Job drawing, mm, ordinate dimensions from the low corner. One solid piece. A direction names the side the tool comes from. Coordinates: 2 decimals unless noted, no trailing zeros. Write each loop counter-clockwise with the first axis right and the second up, starting at its lowest first coordinate (ties: lowest second). Pieces come first, ordered by that corner, then holes. Notation, with made-up numbers: (29, 54) - (49, 54) arc R14 ccw to (49, 78) - close; hole circle Ø4 at (36, 24.5). An arc over 180 degrees is marked (long way). Put each result on its own line as item: value. Start each with the question number.
1. Saw through at D-D, the plane y = 2.5. Write the cut outline in (x, z).
2. Drop flat-ended pins along their axis: P1, Ø3.5, axis at x = 12, y = 5.5, coming from the +Z side; P2, Ø2.5, axis at y = 5.5, z = 12, coming from the -X side; P3, Ø2, axis at y = 4, z = 12, coming from the +X side. Give the stop position or say it passes through.
3. Drill centre lines: L1, parallel to Y at x = 2.3, z = 12; L2, parallel to Z at x = 2.15, y = 5.5. Where is each one in solid material? Low to high. Write a range as from..to.
4. Saw through at B-B, the plane z = 12. Write the cut outline in (x, y), plus the area to 3 significant figures.
5. Saw through at A-A, the plane x = 12. Write the cut outline in (y, z).
6. Pull direction Y, two halves, no side cores. Call the marked faces 3, 4 and 5: released by +Y, released by -Y, zero draft, split by the parting line, or undercut.
7. Which spindle directions (+Z, -Z, +X, -X, +Y, -Y) get a long thin tool onto all of the face, cutting with end or side? Do the marked faces 1 and 2. Say none if no direction does.
8. Saw through at C-C, the plane z = 3.25. Write the cut outline in (x, y), plus the area to 3 significant figures.
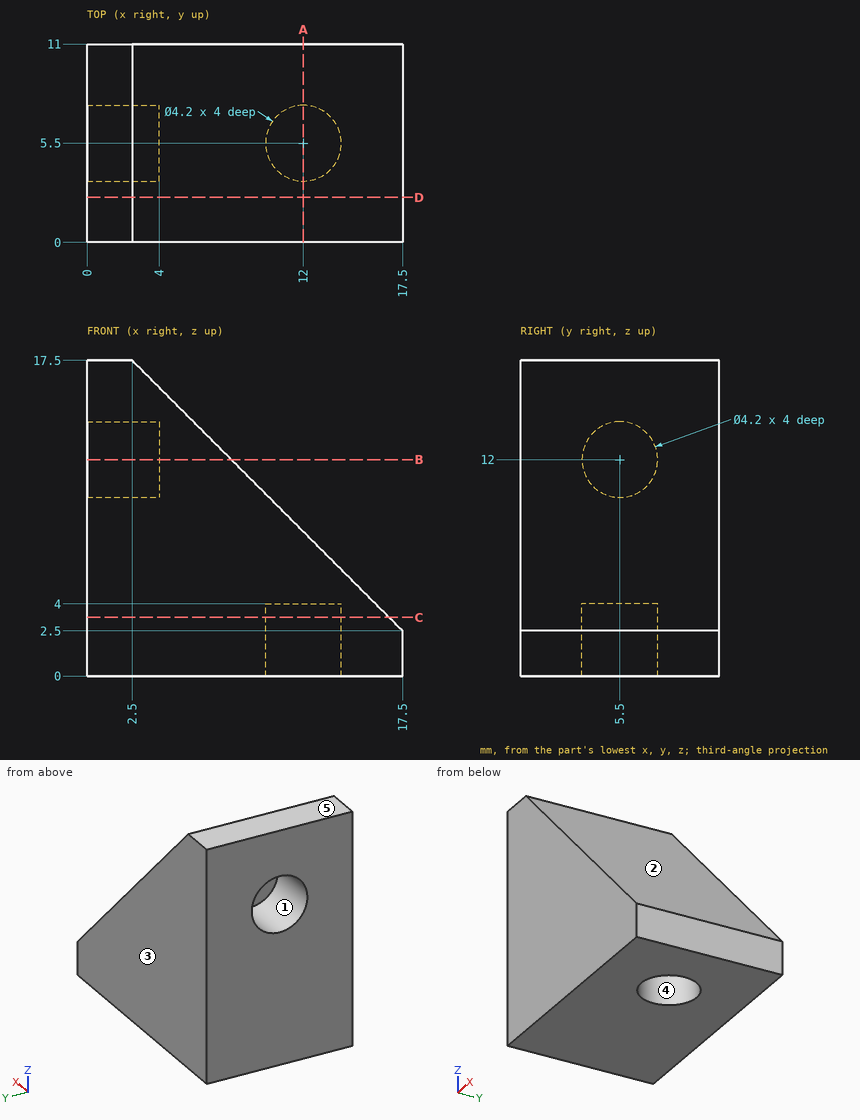
Final values:
1. outline: (0, 0) - (17.5, 0) - (17.5, 2.5) - (2.5, 17.5) - (0, 17.5) - close
2. P1: stops at z = 9.75
2. P2: stops at x = 4
2. P3: stops at x = 9
3. L1: y = 0..3.4, 7.6..11
3. L2: z = 0..9.9, 14.1..17.5
4. outline: (0, 0) - (8, 0) - (8, 11) - (0, 11) - (0, 7.6) - (4, 7.6) - (4, 3.4) - (0, 3.4) - close
4. area: 71.2 mm²
5. outline: (0, 0) - (3.4, 0) - (3.4, 4) - (7.6, 4) - (7.6, 0) - (11, 0) - (11, 8) - (0, 8) - close
6. face 3: released by +Y
6. face 4: undercut
6. face 5: zero draft
7. face 1: -X
7. face 2: +Z, +X, +Y, -Y
8. outline: (0, 0) - (16.75, 0) - (16.75, 11) - (0, 11) - close; hole circle Ø4.2 at (12, 5.5)
8. area: 170 mm²
